from build123d import *

# Parameters (mm, degrees)
BOSS_EXTRUDE1_DEPTH     = 12.7
CUT_EXTRUDE1_DEPTH      = 270.19769127
SKETCH3_W               = 29.1
SKETCH3_H               = 12.7
F_12_CLEARANCE_HOLE1_D  = 6
F_8_CLEARANCE_HOLE1_D   = 4.5
F_1_4_CLEARANCE_HOLE1_D = 6.6
SKETCH10_W              = 2.5
SKETCH10_H              = 36.4125
HOLE1_D                 = 6.4
HOLE1_DEPTH             = 64.36393101
HOLE1_CBORE_D           = 11.2
HOLE1_CBORE_DEPTH       = 11.77643101
CHAMFER1_SIZE           = 3


with BuildPart() as part:
    # Sketch1 → Boss-Extrude1 (new body)
    with BuildSketch(Plane(origin=(0, 0, 0), x_dir=(-1, 0, 0), z_dir=(0, 0, -1))):
        with BuildLine():
            Line((129.246532787, 74.570537656), (211.469455465, 46.304993078))
            Line((211.469455465, 46.304993078), (224.169455465, 46.304993078))
            Line((224.169455465, 46.304993078), (224.169455465, 127.72254562))
            Line((224.169455465, 127.72254562), (151.435240745, 147.211619716))
            ThreePointArc((151.435240745, 147.211619716), (105.257753851, 121.607458019), (129.246532787, 74.570537656))
        make_face()
    extrude(amount=-BOSS_EXTRUDE1_DEPTH)

    # Sketch2 → Cut-Extrude1 (cut, through all)
    with BuildSketch(Plane.XY.offset(12.7)):
        with BuildLine():
            Line((-103.633291463, 112.093938317), (-113.069248332, 112.093938317))
            ThreePointArc((-113.069248332, 112.093938317), (-113.025117032, 110.506438317), (-113.069248332, 108.918938317))
            Line((-113.069248332, 108.918938317), (-103.633291463, 108.918938317))
            ThreePointArc((-103.633291463, 108.918938317), (-103.600117032, 110.506438317), (-103.633291463, 112.093938317))
        make_face()
    extrude(amount=-CUT_EXTRUDE1_DEPTH, mode=Mode.SUBTRACT)

    # Sketch3 → Cut-Revolve1 (revolve, cut)
    with BuildSketch(Plane.XZ.offset(-110.506438317)):
        with Locations((-127.050117032, 6.35)):
            Rectangle(SKETCH3_W, SKETCH3_H)
    revolve(axis=Axis((-141.600117032, 110.506438317, 12.7), (0, 0, -1)), mode=Mode.SUBTRACT)

    # #12 Clearance Hole1 (through all)
    with Locations(Plane.XY.offset(12.7)):
        with Locations((-192.169455465, 89.72254562)):
            Hole(F_12_CLEARANCE_HOLE1_D / 2)

    # #8 Clearance Hole1 (through all)
    with Locations(Plane.XY.offset(12.7)):
        with Locations((-117.978117032, 86.884438317), (-165.222117032, 86.884438317), (-165.222117032, 134.128438317), (-117.978117032, 134.128438317)):
            Hole(F_8_CLEARANCE_HOLE1_D / 2)

    # 1/4 Clearance Hole1 (through all)
    with Locations(Plane(origin=(0, 0, 0), x_dir=(-1, 0, 0), z_dir=(0, 0, -1))):
        with Locations((217.819455465, 53.304993078), (217.819455465, 76.304993078), (217.819455465, 99.304993078)):
            Hole(F_1_4_CLEARANCE_HOLE1_D / 2)

    # Sketch10 → #10 Clearance Hole1 (revolve, cut)
    with BuildSketch(Plane(origin=(-108.633291463, 112.093938317, 6.35), x_dir=(0, 0, -1), z_dir=(1, 0, 0))):
        with Locations((1.25, 18.20625)):
            Rectangle(SKETCH10_W, SKETCH10_H)
    revolve(axis=Axis((-108.633291463, 105.743938317, 6.35), (0, 1, 0)), mode=Mode.SUBTRACT)

    # Hole1
    with Locations(Plane(origin=(0, 84.142507307, 0), x_dir=(-1, 0, 0), z_dir=(0, -1, 0))):
        with Locations((108.633291463, -6.35)):
            CounterBoreHole(HOLE1_D / 2, HOLE1_CBORE_D / 2, HOLE1_CBORE_DEPTH, depth=HOLE1_DEPTH)

    # Chamfer1
    chamfer1_edges = [part.edges().sort_by_distance(p)[0] for p in [
        (-221.119455465, 99.304993078, 0),
        (-221.119455465, 76.304993078, 0),
        (-221.119455465, 53.304993078, 0),
    ]]
    chamfer(chamfer1_edges, length=CHAMFER1_SIZE)


solid = part.part
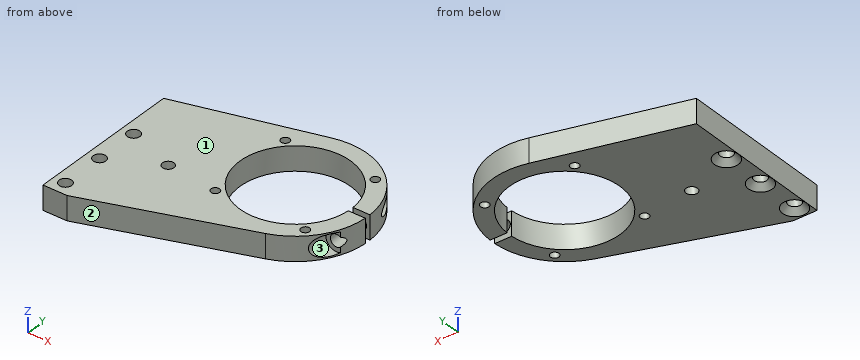
Here's how the part is built. I have some questions about the finished solid (model axes, mm). Face numbers are marked on the shaded views. Round coordinates to 2 decimals unless told otherwise and drop trailing zeros. Loops run counter-clockwise (first coordinate to the right, second up) from the corner with the lowest first, then second, coordinate; pieces in that order, holes last. Notation, with made-up numbers: M -34,82 L 20,82 A11 ccw 20,97 Z; hole C 77.5,18 d1. An arc over 180 degrees is marked long. Write each question's results on one line, items separated by ' | '. Start each with the question number.
(1) I want a section at B-B (x = -192). Please give me the cut outline in (y, z), then the cut area to 3 significant figures.
(2) I want a section at C-C (y = 118). Please give me the cut outline in (x, z), then the cut area to 3 significant figures.
(3) I want a section at A-A (z = 6.35). State how many separate pieces and enclosed holes the cut face has, then the cut area to 3 significant figures.
(4) I want a section at D-D (x = -135). Please give me the cut outline in (y, z).
(5) Thinking about a two-plate mould opening in Z: for the marked faces 1, 2 and 3, which applies, pulls with the +Z half, pulls with the -Z half, needs draft (parallel to the pull), parting line crosses it, or undercut?
(6) Will these pins go through, and if not, where does the flat tip stop? P1, Ø7.5, axis at x = -108.63, z = 6.35, coming from the +Y side; P2, Ø1, axis at x = -166.5, z = 4, coming from the -Y side; P3, Ø2, axis at x = -178, z = 10.5, coming from the -Y side.
(7) If I drill on probe 1 along Y at (x, z) = (-217, 7.5) (3 decimals); probe 2 along X at (y, z) = (101, 6.25); probe 3 along Y at (x, z) = (-149.5, 2), over which ranges is the centre line in solid material (lowest first)? Write a range as from..to.
Solved:
1) outline: M 53,0 L 86.73,0 L 86.73,12.7 L 53,12.7 Z; M 92.72,0 L 136.34,0 L 136.34,12.7 L 92.72,12.7 Z | area: 982 mm²
2) outline: M -224.17,0 L -169.72,0 L -169.72,12.7 L -224.17,12.7 Z; M -113.48,0 L -104.35,0 L -104.35,12.7 L -113.48,12.7 Z; hole C -108.63,6.35 d6.4 | area: 775 mm²
3) separate pieces: 3 | enclosed holes: 8 | area: 5,950 mm²
4) outline: M 72.59,0 L 82.16,0 L 82.16,12.7 L 72.59,12.7 Z; M 138.85,0 L 147.93,0 L 147.93,12.7 L 138.85,12.7 Z
5) face 1: pulls with the +Z half | face 2: needs draft | face 3: undercut
6) P1: stops at y = 134.8 | P2: stops at y = 61.59 | P3: stops at y = 57.47
7) probe 1: y = 46.305..50.108, 56.502..73.108, 79.502..96.108, 102.502..129.644 | probe 2: x = -224.17..-220.65, -214.99..-169.1, -114.1..-111.83, -105.43..-104.81 | probe 3: y = 67.61..82.5, 138.51..147.68
